Autodesk Inventor part; units mm, degrees
ref_plane "YZ Plane" through (0, 0, 0) normal (1, 0, 0) x (0, 1, 0)
ref_plane "XZ Plane" through (0, 0, 0) normal (0, 1, 0) x (-1, 0, 0)
ref_plane "XY Plane" through (0, 0, 0) normal (0, 0, 1) x (1, 0, 0)
sketch "Sketch1" plane through (0, 0, 0) normal (0, 1, 0) x (-1, 0, 0)
  line L0 (0, 0) -> (-20.32, 0)
  line L1 (-20.32, 0) -> (-20.32, -76.2)
  line L2 (-20.32, -76.2) -> (0, -76.2)
  line L3 (0, -76.2) -> (0, 0)
  dimension "d0" = 20.32
  dimension "d1" = 76.2
extrude "Extrusion1" add sketch "Sketch1" along normal blind 7.62
sketch "Sketch2" plane through (0, 7.62, 0) normal (0, 1, 0) x (1, 0, 0)
  line L0 (0, 0) -> (0, 12.7)
  line L1 (0, 12.7) -> (20.32, 12.7)
  line L2 (20.32, 12.7) -> (20.32, 63.5)
  line L3 (20.32, 63.5) -> (0, 63.5)
  line L4 (0, 63.5) -> (0, 12.7)
  dimension "d4" = 12.7
  dimension "d5" = 20.32
  dimension "d6" = 50.8
extrude "Extrusion2" add sketch "Sketch2" along normal blind 43.18
sketch "Sketch3" plane through (20.32, 0, 0) normal (1, 0, 0) x (0, 0, -1)
  line L0 (12.7, 50.8) -> (63.5, 50.8)
  line L1 (38.1, 50.8) -> (38.1, 25.4)
  circle A0 centre (38.1, 25.4) radius 19.05
  point P0 (0, 0)
  dimension "d9" = 25.4
  dimension "d10" = 38.1
extrude "Extrusion3" cut sketch "Sketch3" against normal blind 15.24
fillet "Fillet1" radius 25.4 2 edges at (10.16, 50.8, -63.5) (10.16, 50.8, -12.7)
sketch "Sketch6" plane through (0, 7.62, 0) normal (0, 1, 0) x (1, 0, 0)
  line L0 (0, 0) -> (20.32, 0)
  line L1 (10.16, 0) -> (10.16, 6.35)
  line L2 (20.32, 76.2) -> (0, 76.2)
  line L3 (10.16, 76.2) -> (10.16, 69.85)
  dimension "d20" = 6.35
  dimension "d21" = 6.35
fillet "Fillet2" radius 25.4 2 edges at (10.16, 7.62, -63.5) (10.16, 7.62, -12.7)
hole "Hole1" at (10.16, 7.62, -6.35) at (10.16, 7.62, -69.85) direction (0, -1, 0) diameter 5.08 end through all counterbore diameter 10.16 counterbore depth 3.81
sketch "Sketch7" plane through (10.16, 7.62, -6.35) normal (0, -1, 0) x (1, 0, 0)
  circle A0 centre (0, 0) radius 5.08
  circle A1 centre (0, -63.5) radius 2.54
  line L0 (-2.54, -63.5) -> (0, -63.5)
  circle A2 centre (0, -63.5) radius 5.08
  point P0 (-10.16, 6.35)
  dimension "d30" = 10.16
  dimension "d31" = 10.16
extrude "Extrusion5" cut sketch "Sketch7" against normal blind 15.24 contours A0 | A1 | A2
sketch "Sketch9" plane through (5.08, 25.4, -38.1) normal (1, 0, 0) x (0, 0, -1)
  line L0 (0, 0) -> (0, -6.604)
  circle A0 centre (0, -6.604) radius 6.604
  line L1 (0, -6.604) -> (-3.302, -12.3232)
  line L2 (0, -6.604) -> (6.604, -6.604) construction
  line L3 (0, -6.604) -> (3.302, -12.3232)
  line L4 (0, -6.604) -> (6.604, -6.604) construction
  line L5 (-3.302, -12.3232) -> (-4.064, -13.6431)
  line L6 (3.302, -12.3232) -> (4.064, -13.6431)
  line L7 (3.302, -12.3232) -> (4.826, -12.3232) construction
  circle A1 centre (-4.064, -13.6431) radius 1.778
  circle A2 centre (4.064, -13.6431) radius 1.778
  circle A3 centre (0, 0) radius 19.05
  line L8 (-19.05, 0) -> (-17.526, 0)
  line L9 (-17.526, 0) -> (-15.875, 0)
  circle A4 centre (-15.875, 0) radius 1.651
  line L10 (19.05, 0) -> (17.526, 0)
  line L11 (17.526, 0) -> (15.875, 0)
  circle A5 centre (15.875, 0) radius 1.651
  line L12 (0, 0) -> (-9.525, 16.4978)
  line L13 (0, 0) -> (9.525, 16.4978)
  line L14 (-9.525, 16.4978) -> (-8.763, 15.178)
  line L15 (-8.763, 15.178) -> (-7.9375, 13.7482)
  line L16 (9.525, 16.4978) -> (8.763, 15.178)
  line L17 (8.763, 15.178) -> (7.9375, 13.7482)
  circle A6 centre (-7.9375, 13.7482) radius 1.651
  circle A7 centre (7.9375, 13.7482) radius 1.651
  point P0 (-38.1, -25.4)
  point P1 (-2.5627, -12.6905)
  point P2 (2.5627, -12.6905)
  point P3 (3.9897, -11.8666)
  point P4 (-3.9897, -11.8666)
  dimension "d47" = 6.604
  dimension "d48" = 120
  dimension "d49" = 60
  dimension "d50" = 1.524
  dimension "d51" = 1.524
  dimension "d52" = 60
  dimension "d53" = 3.556
  dimension "d54" = 3.556
  dimension "d55" = 1.524
  dimension "d56" = 1.651
  dimension "d57" = 1.524
  dimension "d58" = 1.651
  dimension "d59" = 1.524
  dimension "d60" = 1.651
  dimension "d61" = 1.524
  dimension "d62" = 1.651
extrude "Extrusion7" cut sketch "Sketch9" against normal blind 25.4 contours A0 A2 L3 L0 | L0 L1 A1 A0 | L3 A2 A0 A1 L1 | A1 L1 A0 | A0 A1 | A6 L12 | L12 A6 | A7 L13 | L13 A7 | A1 A0 L1 | A2 A0 L3 | L3 A0 A2 | A2 A0 | A4 | A5
sketch "Sketch10" plane through (5.08, 25.4, -38.1) normal (1, 0, 0) x (0, 0, -1)
  arc A0 (3.9897, -11.8666) -> (-3.9897, -11.8666) centre (0, -6.604) ccw
  circle A1 centre (0, 0) radius 20.1518
  circle A2 centre (0, 0) radius 57.3764
  point P0 (-38.1, -25.4)
extrude "Extrusion8" cut sketch "Sketch10" along normal mid plane 50.8
sketch "Sketch11" plane through (5.08, 25.4, -38.1) normal (1, 0, 0) x (0, 0, -1)
  arc A0 (3.9897, -11.8666) -> (-3.9897, -11.8666) centre (0, -6.604) ccw
  circle A1 centre (0, 0) radius 19.05
  point P0 (-38.1, -25.4)
extrude "Extrusion9" cut sketch "Sketch11" against normal blind 3.81
sketch "Sketch12" plane through (20.32, 25.4, -38.1) normal (1, 0, 0) x (0, 0, -1)
  arc A0 (3.9897, -11.8666) -> (-3.9897, -11.8666) centre (0, -6.604) ccw
  circle A1 centre (0, 0) radius 21.629
  point P0 (-38.1, -25.4)
extrude "Extrusion10" cut sketch "Sketch12" against normal blind 15.24
properties part number "Motor Mount V2"
Read the model definition and answer for the solid it produces. Units are mm, in the model's axes. A direction names the side the tool comes from. Give positions to 0.01 mm unless a question says otherwise; leave off trailing zeros. Order: outer loops, then holes, each group sorted by start corner. A loop starts at its lowest first (then second) coordinate and runs counter-clockwise, first axis right, second up.
(1) Find section C-C (x = 3). Give the vertices of the cut face in (y, z), plus the area to 3 significant figures.
(2) Straight lines are drawn through the part: L1, parallel to Y at x = 0.4, z = -43.5; L2, parallel to Y at x = 2.45, z = -38.1; L3, parallel to Z at x = 0.6, y = 11.5. For each, find the intervals that lie inside material, in ascending order.
(3) Given pin 1 (4 mm diameter, centred on y = 11.76, z = -34.04, fed in from -X); pin 2 (1 mm diameter, centred on x = 2, z = -54, fed in from +Y); pin 3 (2 mm diameter, centred on x = 0.5, z = -35.5, fed in from -Y); pin 4 (2 mm diameter, centred on x = 1, y = 30, fed in from +Z), each flat-ended and moving along its own axis, determine where each tip first touches the part or whether it passes through.
(4) Find section D-D (z = -33). Give the vertices of the cut face in (x, y).
(5) Find section B-B (y = 26.5). Give the vertices of the cut face in (x, z), plus the area to 3 significant figures.
(6) For faces 4 (the cylindrical face through (0.644, 12.192, -38.063)), 5 (the cylindrical face through (3.202, 6.803, -33.97)), 6 (the flat face through (5.08, 7.6, -45.5)), determine the directions among +Z, -Z, +X, -X, +Y, -Y from which every point of the face is accessible in a straight line to the end or side of a thin tool.
(7) Find section A-A (z = -38.1). Give the vertices of the cut face in (x, y), plus the area to 3 significant figures.
(8) For a pull along Y with two mould halves and no side action, classify faces 1 (the cylindrical face through (2.576, 5.727, -33.731)), 2 (the flat face through (0, 30, -38)), 3 (the cylindrical face through (0.644, 26.792, -54.863)) as released by +Y, released by -Y, zero draft, split by the parting line, or undercut.
Result sheet:
1. outline: circle Ø40.3 at (25.4, -38.1); hole circle Ø38.1 at (25.4, -38.1)
1. area: 136 mm2
2. L1: y = 5.99 to 10.58, 12.93 to 14.99, 22.6 to 44.81
2. L2: y = 5.25 to 6.35, 44.45 to 45.55
2. L3: z = -52.69 to -43.92, -40.4 to -35.8, -32.28 to -23.51
3. pin 1: stops at x = 0
3. pin 2: stops at y = 38.4
3. pin 3: stops at y = 5.31
3. pin 4: stops at z = -18.27
4. outline: (0, 5.9) - (5.08, 5.9) - (5.08, 7.05) - (1.27, 7.05) - (1.27, 10.31) - (0, 10.31) - close; (0, 13.2) - (1.27, 13.2) - (1.27, 14.6) - (0, 14.6) - close; (0, 22.99) - (1.27, 22.99) - (1.27, 43.75) - (5.08, 43.75) - (5.08, 44.9) - (0, 44.9) - close
5. outline: (0, -58.22) - (5.08, -58.22) - (5.08, -57.12) - (1.27, -57.12) - (1.27, -55.21) - (0, -55.21) - close; (0, -52.74) - (1.27, -52.74) - (1.27, -23.46) - (0, -23.46) - close; (0, -20.99) - (1.27, -20.99) - (1.27, -19.08) - (5.08, -19.08) - (5.08, -17.98) - (0, -17.98) - close
5. area: 53.3 mm2
6. face 4: +X, -X
6. face 5: +X
6. face 6: +Z, -Z, +X, +Y, -Y
7. outline: (0, 5.25) - (5.08, 5.25) - (5.08, 6.35) - (1.27, 6.35) - (1.27, 12.19) - (0, 12.19) - close; (0, 25.4) - (1.27, 25.4) - (1.27, 44.45) - (5.08, 44.45) - (5.08, 45.55) - (0, 45.55) - close
7. area: 42.8 mm2
8. face 1: split by the parting line
8. face 2: zero draft
8. face 3: undercut
